Work out the finished part from the listing and answer in its coordinate system (mm). Round coordinates to 2 decimals unless told otherwise and drop trailing zeros. Order: outer loops, then holes, each group sorted by start corner. A loop starts at its lowest first (then second) coordinate and runs counter-clockwise, first axis right, second up. Notation, with made-up numbers: (60.25, 8) - (80.25, 8) arc R17 cw to (80.25, 15) - close; hole circle Ø5 at (46, 7.25). An arc over 180 degrees is marked (long way). Use CSV: the item, a comma, the result in double quotes.
from build123d import *

# Parameters (mm, degrees)
F0_R     = 50.8
F0_R_2   = 38.1
F1_DEPTH = 12.7
F2_R     = 3.175
F3_DEPTH = 12.7


with BuildPart() as f1:
    # F0 (on Front) → F1 (new body)
    with BuildSketch(Plane.XZ):
        Circle(F0_R)
        Circle(F0_R_2, mode=Mode.SUBTRACT)
    extrude(amount=F1_DEPTH)

    # F2 (on face) → F3 (cut)
    with BuildSketch(Plane.XZ.offset(12.7)):
        with Locations((-19.05, 38.1)):
            Circle(F2_R)
        with Locations((19.05, 38.1)):
            Circle(F2_R)
        with Locations((19.05, -38.1)):
            Circle(F2_R)
        with Locations((-19.05, -38.1)):
            Circle(F2_R)
    extrude(amount=-F3_DEPTH, mode=Mode.SUBTRACT)


solid = f1.part
(1) Find section B-B (z = 0). Determine the outline of the cut face in (x, y).
Findings below:
outline,"(-50.8, -12.7) - (-38.1, -12.7) - (-38.1, 0) - (-50.8, 0) - close; (38.1, -12.7) - (50.8, -12.7) - (50.8, 0) - (38.1, 0) - close"
(2) Find section C-C (z = 40). Determine the outline of the cut face in (x, y).
Findings below:
outline,"(-31.32, -12.7) - (-21.59, -12.7) - (-21.59, 0) - (-31.32, 0) - close; (-16.51, -12.7) - (16.51, -12.7) - (16.51, 0) - (-16.51, 0) - close; (21.59, -12.7) - (31.32, -12.7) - (31.32, 0) - (21.59, 0) - close"
(3) Find section D-D (x = -19.05). Determine the outline of the cut face in (y, z) (3 decimals), and give its area (3 significant figures).
Findings below:
outline,"(-12.7, -47.093) - (0, -47.093) - (0, -41.275) - (-12.7, -41.275) - close; (-12.7, -34.925) - (0, -34.925) - (0, -32.996) - (-12.7, -32.996) - close; (-12.7, 32.996) - (0, 32.996) - (0, 34.925) - (-12.7, 34.925) - close; (-12.7, 41.275) - (0, 41.275) - (0, 47.093) - (-12.7, 47.093) - close"
area,"197 mm²"
(4) Find section A-A (x = 0). Determine the outline of the cut face in (y, z).
Findings below:
outline,"(-12.7, -50.8) - (0, -50.8) - (0, -38.1) - (-12.7, -38.1) - close; (-12.7, 38.1) - (0, 38.1) - (0, 50.8) - (-12.7, 50.8) - close"
(5) Find the intervals of material crossed by L1, parallel to Z at x = 0, y = -4.5; L2, parallel to Z at x = -19.05, y = -7.25 (3 decimals); L3, parallel to Z at x = -2.5, y = -11.5, in increasing order. Write a range as from..to.
Findings below:
L1,"z = -50.8..-38.1, 38.1..50.8"
L2,"z = -47.093..-41.275, -34.925..-32.996, 32.996..34.925, 41.275..47.093"
L3,"z = -50.74..-38.02, 38.02..50.74"
(6) The mould has two halves that part along Z. Classify faces 1 (the flat face through (7, -12.7, 38)), 2 (the cylindrical face through (-11.012, -6.261, -49.592)), 3 (the cylindrical face through (-30.235, -6.261, -23.183)): released by +Z, released by -Z, zero draft, split by the parting line, or undercut.
Findings below:
face 1,"zero draft"
face 2,"split by the parting line"
face 3,"undercut"
(7) Each of these flat-tipped pins is pushed along its axis until it touches: pin 1 (5 mm diameter, centred on x = 28, y = -11, fed in from +Z); pin 2 (2 mm diameter, centred on y = -5.5, z = -2.5, fed in from +X); pin 3 (6 mm diameter, centred on x = 18, y = -9, fed in from -Z); pin 4 (4 mm diameter, centred on x = 19.05, z = -38.1, fed in from +Y). Where does it stop, or does it pass through?
Findings below:
pin 1,"stops at z = 43.94"
pin 2,"stops at x = 50.78"
pin 3,"stops at z = -48.53"
pin 4,"passes through"
